Autodesk Inventor part; units mm, degrees
ref_plane "YZ Plane" through (0, 0, 0) normal (1, 0, 0) x (0, 1, 0)
ref_plane "XZ Plane" through (0, 0, 0) normal (0, 1, 0) x (-1, 0, 0)
ref_plane "XY Plane" through (0, 0, 0) normal (0, 0, 1) x (1, 0, 0)
sketch "Sketch1" plane through (0, 0, 0) normal (0, 0, 1) x (1, 0, 0)
  circle A0 centre (0, 0) radius 12.7
  dimension "d0" = 25.4
extrude "Extrusion1" add sketch "Sketch1" along normal blind 1.5875
sketch "Sketch2" plane through (0, 0, 1.5875) normal (0, 0, 1) x (1, 0, 0)
  circle A0 centre (0, 0) radius 3.175
  dimension "d3" = 6.35
extrude "Extrusion2" add sketch "Sketch2" along normal blind 6.35
sketch "Sketch3" plane through (0, 0, 7.9375) normal (0, 0, 1) x (1, 0, 0)
  circle A0 centre (0, 0) radius 12.7
  dimension "d6" = 25.4
extrude "Extrusion3" add sketch "Sketch3" along normal blind 1.5875
sketch "Sketch4" plane through (0, 0, 9.525) normal (0, 0, 1) x (1, 0, 0)
  circle A0 centre (0, 0) radius 3.175
  dimension "d9" = 6.35
extrude "Extrusion4" add sketch "Sketch4" along normal blind 6.35
sketch "Sketch5" plane through (0, 0, 15.875) normal (0, 0, 1) x (1, 0, 0)
  circle A0 centre (0, 0) radius 12.7
  dimension "d12" = 25.4
extrude "Extrusion5" add sketch "Sketch5" along normal blind 1.5875
equation "\"d0\" = spoolD"
equation "\"d1\" = spoolT"
equation "\"d3\" = hubD"
equation "\"d4\" = hubH"
equation "\"d6\" = spoolD"
equation "\"d7\" = spoolT"
equation "\"d9\" = hubD"
equation "\"d10\" = hubH"
equation "\"d12\" = spoolD"
equation "\"d13\" = spoolT"
equation "\"spoolD\" = 25.4"
equation "\"hubD\" = 6.35"
equation "\"spoolT\" = 1.5875"
equation "\"hubH\" = 6.35"
equation "\"hornT\" = 1.5875"
equation "\"hornD\" = 25.4"
equation "\"hornS\" = 2.794"
equation "\"hornOD\" = 8.89"
equation "\"hornH\" = 2.54"
equation "\"hornID\" = 6.096"
equation "\"inset\" = 2.032"
equation "\"insetD\" = 5.842"
equation "\"servW\" = 20.1168"
equation "\"servL\" = 40.5892"
equation "\"servML\" = 49.784"
equation "\"servMW\" = 10.033"
equation "\"servMD\" = 3.175"
equation "\"housL\" = 53.975"
equation "\"housW\" = 28.575"
equation "\"housT\" = 2.54"
equation "\"housBT\" = 1.5875"
equation "\"housH\" = 39.116"
equation "\"guideW\" = 9.144"
equation "\"guideH\" = 23.114"
equation "\"guideD\" = 3.175"
properties part number "Spool"
The model under review builds one solid part; all positions refer to its coordinate system, in mm. A direction names the side the tool comes from. Coordinates: 2 decimals unless noted, no trailing zeros. Order: outer loops, then holes, each group sorted by start corner. A loop starts at its lowest first (then second) coordinate and runs counter-clockwise, first axis right, second up. Notation, with made-up numbers: (-11, 30.25) -> (5, 30.25) arc R16 cw to (5, 43.25) -> close; hole circle Ø1 at (10, 73.25). An arc over 180 degrees is marked (long way). Answer in a Markdown table with one row per item.
(1) Wall thickness on line 1 along Z through (x, y) = (-5, -5) (1 decimal); line 2 along Y through (x, z) = (0.75, 16); line 3 along Y through (x, z) = (-10.5, 9.25): over which ranges is each line inside the solid? List them lowest first.
Answers:
| item | result |
|---|---|
| line 1 | 0 to 1.6, 7.9 to 9.5, 15.9 to 17.5 |
| line 2 | -12.68 to 12.68 |
| line 3 | -7.14 to 7.14 |
(2) Consider section B-B (x = -3.5). Write out the cut boundary in (y, z) (1 decimal), plus the area to 3 significant figures.
Answers:
| item | result |
|---|---|
| outline | (-12.2, 0) -> (12.2, 0) -> (12.2, 1.6) -> (-12.2, 1.6) -> close; (-12.2, 7.9) -> (12.2, 7.9) -> (12.2, 9.5) -> (-12.2, 9.5) -> close; (-12.2, 15.9) -> (12.2, 15.9) -> (12.2, 17.5) -> (-12.2, 17.5) -> close |
| area | 116 mm² |
(3) The part is to be moulded in two halves that separate along Z. For faces 1 (the cylindrical face through (-2.75, 12.4, 8.72)), 2 (the flat face through (0, 0, 0)), 3 (the flat face through (3, -3, 9.525)), 4 (the flat face through (3, -3, 7.938)), say which applies: +Z half, -Z half, draft (parallel to the pull), parting line (faces both ways), or undercut.
Answers:
| item | result |
|---|---|
| face 1 | draft |
| face 2 | -Z half |
| face 3 | undercut |
| face 4 | undercut |
(4) Insertion check: pin 1 (8 mm diameter, centred on y = -7.5, z = 4.5, fed in from +X); pin 2 (8 mm diameter, centred on y = -4.5, z = 8.5, fed in from +X); pin 3 (1.5 mm diameter, centred on y = -9, z = 13.5, fed in from +X); pin 4 (8 mm diameter, centred on y = 4.5, z = 14.5, fed in from -X). Each pin has a flat end and moves straight along its axis. Give the tip position at first contact, or say it passes through.
Answers:
| item | result |
|---|---|
| pin 1 | x = 11.77 |
| pin 2 | x = 12.69 |
| pin 3 | through |
| pin 4 | x = -12.68 |
(5) Consider section A-A (y = 0). Write out the cut boundary in (x, z) (1 decimal), plus the area to 3 significant figures.
Answers:
| item | result |
|---|---|
| outline | (-12.7, 0) -> (12.7, 0) -> (12.7, 1.6) -> (3.2, 1.6) -> (3.2, 7.9) -> (12.7, 7.9) -> (12.7, 9.5) -> (3.2, 9.5) -> (3.2, 15.9) -> (12.7, 15.9) -> (12.7, 17.5) -> (-12.7, 17.5) -> (-12.7, 15.9) -> (-3.2, 15.9) -> (-3.2, 9.5) -> (-12.7, 9.5) -> (-12.7, 7.9) -> (-3.2, 7.9) -> (-3.2, 1.6) -> (-12.7, 1.6) -> close |
| area | 202 mm² |
(6) Consider section D-D (y = 7.75). Write out the cut boundary in (x, z) (1 decimal), plus the area to 3 significant figures.
Answers:
| item | result |
|---|---|
| outline | (-10.1, 0) -> (10.1, 0) -> (10.1, 1.6) -> (-10.1, 1.6) -> close; (-10.1, 7.9) -> (10.1, 7.9) -> (10.1, 9.5) -> (-10.1, 9.5) -> close; (-10.1, 15.9) -> (10.1, 15.9) -> (10.1, 17.5) -> (-10.1, 17.5) -> close |
| area | 95.8 mm² |
(7) Machinability: for faces 5 (the flat face through (3, -3, 1.588)), 6 (the cylindrical face through (-2.75, 12.4, 16.66)), which of the approach directions +Z, -Z, +X, -X, +Y, -Y give a long, thin tool a straight path to every point of the face, cutting with its end or side? Answer none if there is none.
Answers:
| item | result |
|---|---|
| face 5 | none |
| face 6 | +Z, -Z |
